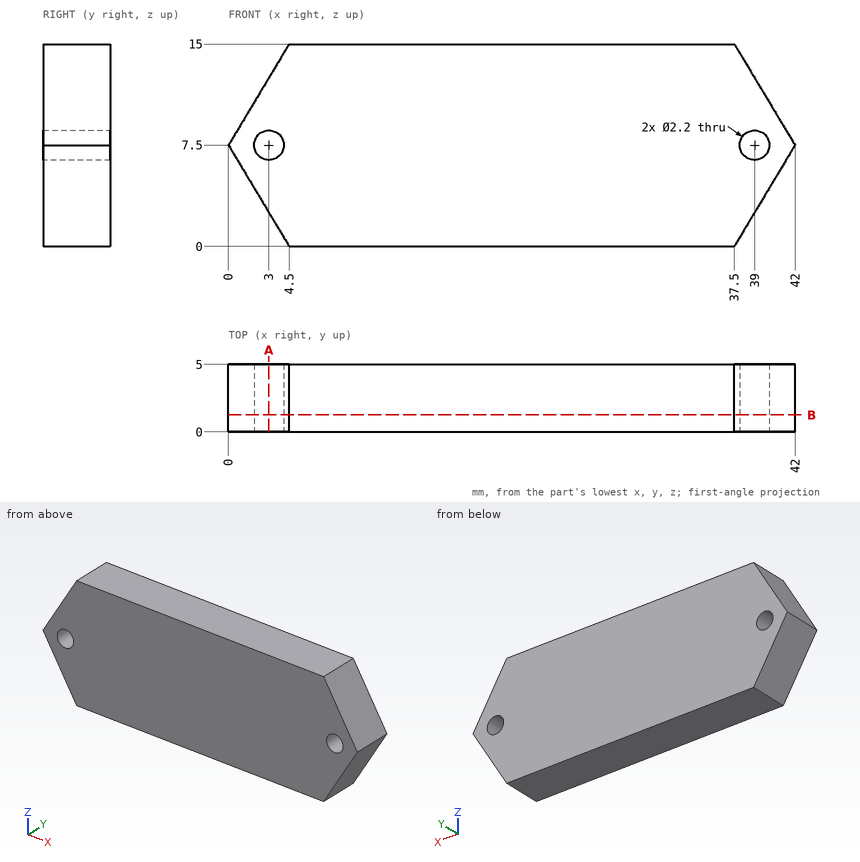
Design review of the part shown in the three views and the two pictorial views. Dimensions are in mm from the part's minimum x, y and z. Round coordinates to 2 decimals unless told otherwise and drop trailing zeros. Write each loop counter-clockwise with the first axis right and the second up, starting at its lowest first coordinate (ties: lowest second). Pieces come first, ordered by that corner, then holes. Notation, with made-up numbers: (62.5, 25.25) -> (90.5, 25.25) arc R20 ccw to (90.5, 33.25) -> close; hole circle Ø9 at (31, 66.25). An arc over 180 degrees is marked (long way). Write item = value, one per line. Start each with the question number.
1) Take a section at A-A, the plane x = 3. State the section outline as (y, z) points, plus the area to 3 significant figures.
2) Clearance check with flat-ended pins moving along their axes: pin 1 (1.8 mm diameter, centred on x = 39, z = 7.5, fed in from +Y); pin 2 (1.5 mm diameter, centred on y = 4, z = 11, fed in from -X). State where each tip first meets the part, or that it passes through.
3) Wall thickness on probe 1 along Z at (x, y) = (2, 0.3); probe 2 along Z at (x, y) = (39, 2.9); probe 3 along X at (y, z) = (2.95, 5.75): over which ranges is each line inside the solid? List them lowest first. Write a range as from..to.
4) Take a section at B-B, the plane y = 1.25. State the section outline as (x, z) points.
Results list:
q1.outline = (0, 2.5) -> (5, 2.5) -> (5, 6.4) -> (0, 6.4) -> close; (0, 8.6) -> (5, 8.6) -> (5, 12.5) -> (0, 12.5) -> close
q1.area = 39.0 mm²
q2.pin_1 = through
q2.pin_2 = 1.65
q3.probe_1 = 4.17..7.04, 7.96..10.83
q3.probe_2 = 2.5..6.4, 8.6..12.5
q3.probe_3 = 1.05..40.95
q4.outline = (0, 7.5) -> (4.5, 0) -> (37.5, 0) -> (42, 7.5) -> (37.5, 15) -> (4.5, 15) -> close; hole circle Ø2.2 at (3, 7.5); hole circle Ø2.2 at (39, 7.5)
